The listing builds one solid part. Answer for the finished solid, in the listing's coordinates (mm). Give positions to 0.01 mm unless a question says otherwise; leave off trailing zeros. Write each loop counter-clockwise with the first axis right and the second up, starting at its lowest first coordinate (ties: lowest second). Pieces come first, ordered by that corner, then holes. Notation, with made-up numbers: M -15.5,49 L -0.5,49 A17 ccw -0.5,73 Z; hole C 77.25,23.5 d6. An arc over 180 degrees is marked long. Return JSON: item names as keys, results as strings.
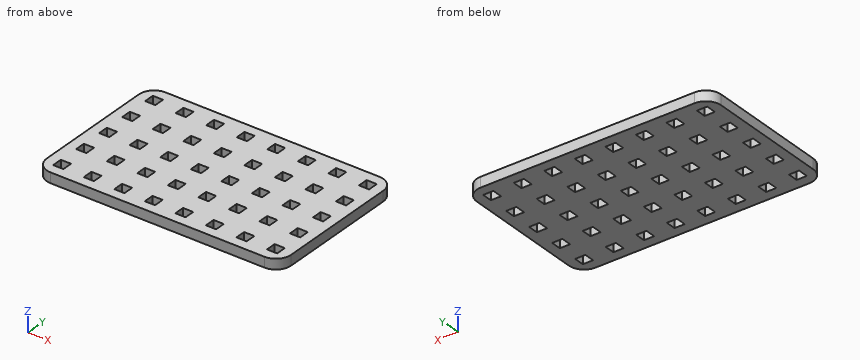
from build123d import *

# Parameters (mm, degrees)
MODEL_W                 = 3
MODEL_H                 = 3
SALIENTE_EXTRUIR1_DEPTH = 3


with BuildPart() as part:
    # Model → Saliente-Extruir1 (new body)
    with BuildSketch(Plane.XY):
        with BuildLine():
            Line((77.4201517, 259.741779533), (77.4201517, 295.741779533))
            ThreePointArc((77.4201517, 295.741779533), (76.102132215, 298.923760049), (72.9201517, 300.241779533))
            Line((72.9201517, 300.241779533), (9.9201517, 300.241779533))
            ThreePointArc((9.9201517, 300.241779533), (6.738171185, 298.923760049), (5.4201517, 295.741779533))
            Line((5.4201517, 295.741779533), (5.4201517, 259.741779533))
            ThreePointArc((5.4201517, 259.741779533), (6.738171185, 256.559799018), (9.9201517, 255.241779533))
            Line((9.9201517, 255.241779533), (72.9201517, 255.241779533))
            ThreePointArc((72.9201517, 255.241779533), (76.102132215, 256.559799018), (77.4201517, 259.741779533))
        make_face()
        with Locations((9.9201517, 295.741779533)):
            Rectangle(MODEL_W, MODEL_H, mode=Mode.SUBTRACT)
        with Locations((18.9201517, 295.741779533)):
            Rectangle(MODEL_W, MODEL_H, mode=Mode.SUBTRACT)
        with Locations((27.9201517, 295.741779533)):
            Rectangle(MODEL_W, MODEL_H, mode=Mode.SUBTRACT)
        with Locations((36.9201517, 295.741779533)):
            Rectangle(MODEL_W, MODEL_H, mode=Mode.SUBTRACT)
        with Locations((45.9201517, 295.741779533)):
            Rectangle(MODEL_W, MODEL_H, mode=Mode.SUBTRACT)
        with Locations((54.9201517, 295.741779533)):
            Rectangle(MODEL_W, MODEL_H, mode=Mode.SUBTRACT)
        with Locations((63.9201517, 295.741779533)):
            Rectangle(MODEL_W, MODEL_H, mode=Mode.SUBTRACT)
        with Locations((72.9201517, 295.741779533)):
            Rectangle(MODEL_W, MODEL_H, mode=Mode.SUBTRACT)
        with Locations((9.9201517, 259.741779533)):
            Rectangle(MODEL_W, MODEL_H, mode=Mode.SUBTRACT)
        with Locations((18.9201517, 259.741779533)):
            Rectangle(MODEL_W, MODEL_H, mode=Mode.SUBTRACT)
        with Locations((27.9201517, 259.741779533)):
            Rectangle(MODEL_W, MODEL_H, mode=Mode.SUBTRACT)
        with Locations((36.9201517, 259.741779533)):
            Rectangle(MODEL_W, MODEL_H, mode=Mode.SUBTRACT)
        with Locations((45.9201517, 259.741779533)):
            Rectangle(MODEL_W, MODEL_H, mode=Mode.SUBTRACT)
        with Locations((54.9201517, 259.741779533)):
            Rectangle(MODEL_W, MODEL_H, mode=Mode.SUBTRACT)
        with Locations((63.9201517, 259.741779533)):
            Rectangle(MODEL_W, MODEL_H, mode=Mode.SUBTRACT)
        with Locations((72.9201517, 259.741779533)):
            Rectangle(MODEL_W, MODEL_H, mode=Mode.SUBTRACT)
        with Locations((72.9201517, 286.741779533)):
            Rectangle(MODEL_W, MODEL_H, mode=Mode.SUBTRACT)
        with Locations((72.9201517, 268.741779533)):
            Rectangle(MODEL_W, MODEL_H, mode=Mode.SUBTRACT)
        with Locations((72.9201517, 277.741779533)):
            Rectangle(MODEL_W, MODEL_H, mode=Mode.SUBTRACT)
        with Locations((9.9201517, 286.741779533)):
            Rectangle(MODEL_W, MODEL_H, mode=Mode.SUBTRACT)
        with Locations((9.9201517, 268.741779533)):
            Rectangle(MODEL_W, MODEL_H, mode=Mode.SUBTRACT)
        with Locations((9.9201517, 277.741779533)):
            Rectangle(MODEL_W, MODEL_H, mode=Mode.SUBTRACT)
        with Locations((18.9201517, 268.741779533)):
            Rectangle(MODEL_W, MODEL_H, mode=Mode.SUBTRACT)
        with Locations((27.9201517, 268.741779533)):
            Rectangle(MODEL_W, MODEL_H, mode=Mode.SUBTRACT)
        with Locations((36.9201517, 268.741779533)):
            Rectangle(MODEL_W, MODEL_H, mode=Mode.SUBTRACT)
        with Locations((63.9201517, 268.741779533)):
            Rectangle(MODEL_W, MODEL_H, mode=Mode.SUBTRACT)
        with Locations((45.9201517, 268.741779533)):
            Rectangle(MODEL_W, MODEL_H, mode=Mode.SUBTRACT)
        with Locations((54.9201517, 268.741779533)):
            Rectangle(MODEL_W, MODEL_H, mode=Mode.SUBTRACT)
        with Locations((18.9201517, 277.741779533)):
            Rectangle(MODEL_W, MODEL_H, mode=Mode.SUBTRACT)
        with Locations((27.9201517, 277.741779533)):
            Rectangle(MODEL_W, MODEL_H, mode=Mode.SUBTRACT)
        with Locations((36.9201517, 277.741779533)):
            Rectangle(MODEL_W, MODEL_H, mode=Mode.SUBTRACT)
        with Locations((63.9201517, 277.741779533)):
            Rectangle(MODEL_W, MODEL_H, mode=Mode.SUBTRACT)
        with Locations((18.9201517, 286.741779533)):
            Rectangle(MODEL_W, MODEL_H, mode=Mode.SUBTRACT)
        with Locations((27.9201517, 286.741779533)):
            Rectangle(MODEL_W, MODEL_H, mode=Mode.SUBTRACT)
        with Locations((36.9201517, 286.741779533)):
            Rectangle(MODEL_W, MODEL_H, mode=Mode.SUBTRACT)
        with Locations((63.9201517, 286.741779533)):
            Rectangle(MODEL_W, MODEL_H, mode=Mode.SUBTRACT)
        with Locations((45.9201517, 277.741779533)):
            Rectangle(MODEL_W, MODEL_H, mode=Mode.SUBTRACT)
        with Locations((54.9201517, 277.741779533)):
            Rectangle(MODEL_W, MODEL_H, mode=Mode.SUBTRACT)
        with Locations((45.9201517, 286.741779533)):
            Rectangle(MODEL_W, MODEL_H, mode=Mode.SUBTRACT)
        with Locations((54.9201517, 286.741779533)):
            Rectangle(MODEL_W, MODEL_H, mode=Mode.SUBTRACT)
    extrude(amount=SALIENTE_EXTRUIR1_DEPTH)


solid = part.part
Item 1: Find the intervals of material crossed by line 1 (Y direction, x = 10.5, z = 0.2); line 2 (X direction, y = 297.5, z = 0.9); line 3 (X direction, y = 257, z = 2.15), in increasing order.
Geometry results:
{"line 1": "y = 255.24 to 258.24, 261.24 to 267.24, 270.24 to 276.24, 279.24 to 285.24, 288.24 to 294.24, 297.24 to 300.24", "line 2": "x = 5.78 to 77.06", "line 3": "x = 6.35 to 76.49"}
Item 2: A cutting plane is placed at A-A, the plane x = 28.5. Write down the section's boundary in (y, z).
Geometry results:
{"outline": "M 255.24,0 L 258.24,0 L 258.24,3 L 255.24,3 Z; M 261.24,0 L 267.24,0 L 267.24,3 L 261.24,3 Z; M 270.24,0 L 276.24,0 L 276.24,3 L 270.24,3 Z; M 279.24,0 L 285.24,0 L 285.24,3 L 279.24,3 Z; M 288.24,0 L 294.24,0 L 294.24,3 L 288.24,3 Z; M 297.24,0 L 300.24,0 L 300.24,3 L 297.24,3 Z"}
Item 3: A cutting plane is placed at B-B, the plane y = 269. Count the separate pieces of the cut face and the enclosed holes in it, plus the area to 3 significant figures.
Geometry results:
{"separate pieces": "9", "enclosed holes": "0", "area": "144 mm2"}
Item 4: Given pin 1 Ø2 at (x, y) = (14, 277.5) entering from -Z, flat-ended and moving along its own axis, determine where the tip first touches the part or whether it passes through.
Geometry results:
{"pin 1": "stops at z = 0"}
